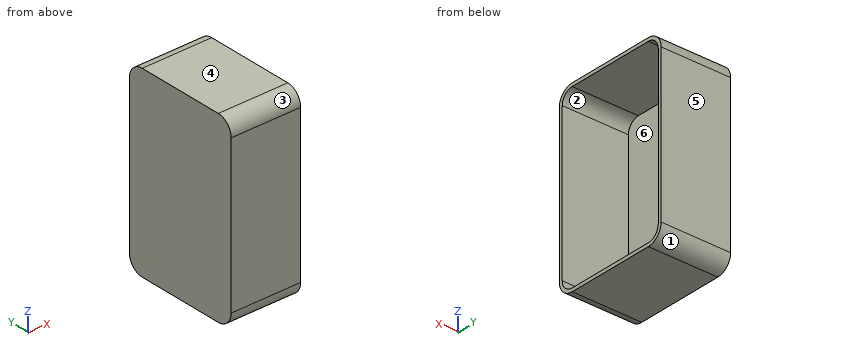
Autodesk Fusion 360 part; units mm, degrees
sketch "Esquisse1" plane through (0, 0, 0) normal (1, 0, 0) x (0, 0, -1)
  line L0 (166.9054, -107.1527) -> (-0.0946, -107.1527)
  circle A0 centre (13.4054, -93.6527) radius 13.5
  line L1 (-0.0946, -107.1527) -> (-0.0946, -0.1527)
  circle A1 centre (13.4054, -13.6527) radius 13.5
  line L2 (-0.0946, -0.1527) -> (166.9054, -0.1527)
  circle A2 centre (153.4054, -13.6527) radius 13.5
  line L3 (166.9054, -0.1527) -> (166.9054, -107.1527)
  circle A3 centre (153.4054, -93.6527) radius 13.5
  dimension "d44" = 107
  dimension "d45" = 167
  dimension "d24" = 27
  dimension "d25" = 27
  dimension "d26" = 27
  dimension "d27" = 27
extrude "Extrusion3" add sketch "Esquisse1" along normal blind 3 contours L0 A0 L1 A1 L2 A2 L3 A3 | A3 | A0 | A2 | A1
sketch "Esquisse3" plane through (3, 0, 0) normal (1, 0, 0) x (0, 0, -1)
  arc A0 (13.4054, -0.1527) -> (-0.0946, -13.6527) centre (13.4054, -13.6527) ccw
  line L0 (-0.0946, -13.6527) -> (-0.0946, -93.6527)
  arc A1 (-0.0946, -93.6527) -> (13.4054, -107.1527) centre (13.4054, -93.6527) ccw
  line L1 (13.4054, -107.1527) -> (153.4054, -107.1527)
  arc A2 (153.4054, -107.1527) -> (166.9054, -93.6527) centre (153.4054, -93.6527) ccw
  line L2 (166.9054, -93.6527) -> (166.9054, -13.6527)
  arc A3 (166.9054, -13.6527) -> (153.4054, -0.1527) centre (153.4054, -13.6527) ccw
  line L3 (153.4054, -0.1527) -> (13.4054, -0.1527)
  line L4 (13.4054, -0.1527) -> (13.4054, -107.1527)
  line L5 (-0.0946, -13.6527) -> (166.9054, -13.6527)
  line L6 (153.4054, -0.1527) -> (153.4054, -107.1527)
  line L7 (166.9054, -93.6527) -> (-0.0946, -93.6527)
  line L8 (13.4054, -3.1527) -> (153.4054, -3.1527)
  line L9 (163.9054, -13.6527) -> (163.9054, -93.6527)
  line L10 (153.4054, -104.1527) -> (13.4054, -104.1527)
  line L11 (2.9054, -93.6527) -> (2.9054, -13.6527)
  line L12 (-0.0946, -0.1527) -> (166.9054, -0.1527)
  line L13 (-0.0946, -107.1527) -> (-0.0946, -0.1527)
  line L14 (166.9054, -107.1527) -> (-0.0946, -107.1527)
  line L15 (166.9054, -0.1527) -> (166.9054, -107.1527)
  arc A4 (13.4054, -3.1527) -> (2.9054, -13.6527) centre (13.4054, -13.6527) ccw
  arc A5 (163.9054, -13.6527) -> (153.4054, -3.1527) centre (153.4054, -13.6527) ccw
  arc A6 (2.9054, -93.6527) -> (13.4054, -104.1527) centre (13.4054, -93.6527) ccw
  arc A7 (153.4054, -104.1527) -> (163.9054, -93.6527) centre (153.4054, -93.6527) ccw
  dimension "d52" = 3
  dimension "d53" = 3
  dimension "d54" = 3
  dimension "d55" = 3
extrude "Extrusion4" add sketch "Esquisse3" along normal blind 60 contours A0 L4 L5 A4 | L3 L4 L6 L8 L12 | L0 L5 L7 L11 L13 | A3 L5 L6 A5 | A1 L4 L7 A6 | L2 L5 L7 L9 L15 | L1 L4 L6 L10 L14 | A2 L6 L7 A7
equation "d10 = largEntrePied + diaPiedBois"
equation "d11 = longEntrePied + diaPiedBois"
equation "d12 = diaPiedBois"
equation "d13 = diaExtPiedBois / 2"
equation "d14 = diaExtPiedBois / 2"
equation "d15 = diaPiedBois"
equation "d16 = diaPiedBois"
equation "d17 = diaPiedBois"
equation "d18 = diaExtPiedBois / 2"
equation "d44 = largEntrePied + diaExtPiedBois"
equation "d45 = longEntrePied + diaExtPiedBois"
equation "d24 = diaPiedBois + 5 mm"
equation "d25 = diaPiedBois + 5 mm"
equation "d26 = diaPiedBois + 5 mm"
equation "d27 = diaPiedBois + 5 mm"
Design review of the part built by this model. Coordinates are the model's own, in mm. Face numbers are marked on the shaded views. A direction names the side the tool comes from. Give positions to 0.01 mm unless a question says otherwise; leave off trailing zeros. Order: outer loops, then holes, each group sorted by start corner. A loop starts at its lowest first (then second) coordinate and runs counter-clockwise, first axis right, second up. Notation, with made-up numbers: (32.25, 27.25) - (88.25, 27.25) arc R23 cw to (88.25, 43.25) - close; hole circle Ø7 at (36, 72.25). An arc over 180 degrees is marked (long way). Write item = value, one per line. Start each with the question number.
Q1. We need section B-B on z = -98.5. State the section outline as (x, y) points, plus the area to 3 significant figures.
Q2. We need section C-C on y = -86.5. State the section outline as (x, z) points.
Q3. Mouldability with a two-part tool opening along Y and no side actions: class the marked faces 3, 4, 5 and 6 as released by +Y, released by -Y, zero draft, split by the parting line, or undercut.
Q4. We need section A-A on x = 22. State the section outline as (y, z) points, plus the area to 3 significant figures.
Q5. To check wall thickness, follow L1, parallel to Y at x = 36.5, z = -62.5; L2, parallel to Z at x = 25, y = -31.5; L3, parallel to X at y = -15.5, z = -22. State the ranges of each line that lie inside material, in increasing order. Write a range as from..to.
Q6. Clearance check with a flat-ended pin moving along its axis: pin 1 Ø12 at (y, z) = (-77.5, -68) entering from +X. State where the tip first meets the part, or that it passes through.
Q7. Tool access review of the marked faces 1 and 2: name each direction out of +Z, -Z, +X, -X, +Y, -Y from which nothing blocks a thin tool from reaching the whole face with its end or side.
Working result:
q1.outline = (0, -107.15) - (63, -107.15) - (63, -104.15) - (3, -104.15) - (3, -3.15) - (63, -3.15) - (63, -0.15) - (0, -0.15) - close
q1.area = 681 mm²
q2.outline = (0, -166.91) - (63, -166.91) - (63, -163.91) - (3, -163.91) - (3, -2.91) - (63, -2.91) - (63, 0.09) - (0, 0.09) - close
q3.face_3 = released by -Y
q3.face_4 = zero draft
q3.face_5 = released by +Y
q3.face_6 = undercut
q4.outline = (-107.15, -153.41) arc R13.5 ccw to (-93.65, -166.91) - (-13.65, -166.91) arc R13.5 ccw to (-0.15, -153.41) - (-0.15, -13.41) arc R13.5 ccw to (-13.65, 0.09) - (-93.65, 0.09) arc R13.5 ccw to (-107.15, -13.41) - close; hole (-104.15, -153.41) arc R10.5 ccw to (-93.65, -163.91) - (-13.65, -163.91) arc R10.5 ccw to (-3.15, -153.41) - (-3.15, -13.41) arc R10.5 ccw to (-13.65, -2.91) - (-93.65, -2.91) arc R10.5 ccw to (-104.15, -13.41) - close
q4.area = 1,550 mm²
q5.L1 = -107.15..-104.15, -3.15..-0.15
q5.L2 = -166.91..-163.91, -2.91..0.09
q5.L3 = 0..3
q6.pin_1 = 3
q7.face_1 = -Z, +X, -X, +Y
q7.face_2 = +X
